```python
from build123d import *

# Parameters (mm, degrees)
SKETCH1_W          = 114.3
SKETCH1_H          = 120.65
EXTRUDE1_DEPTH     = 1.5
SKETCH2_R          = 1.55
SKETCH2_R_2        = 1.5875
CUT_EXTRUDE1_DEPTH = 84.111239463


with BuildPart() as part:
    # Sketch1 → Extrude1 (new body)
    with BuildSketch(Plane.XY):
        Rectangle(SKETCH1_W, SKETCH1_H)
    extrude(amount=EXTRUDE1_DEPTH)

    # Sketch2 → Cut-Extrude1 (cut, through all)
    with BuildSketch(Plane.XY.offset(1.5)):
        with Locations((-53.975, 3.175)):
            Circle(SKETCH2_R)
        with Locations((-47.625, -3.175)):
            Circle(SKETCH2_R)
        with Locations((53.975, 3.175)):
            Circle(SKETCH2_R)
        with Locations((47.625, -3.175)):
            Circle(SKETCH2_R)
        Circle(SKETCH2_R)
        with Locations((-53.18125, 57.15)):
            Circle(SKETCH2_R)
        with Locations((-53.18125, -19.05)):
            Circle(SKETCH2_R)
        with Locations((-53.18125, 38.1)):
            Circle(SKETCH2_R)
        with Locations((-53.18125, 19.05)):
            Circle(SKETCH2_R)
        with Locations((-53.18125, -38.1)):
            Circle(SKETCH2_R)
        with Locations((-53.18125, -57.15)):
            Circle(SKETCH2_R)
        with Locations((53.975, 57.15)):
            Circle(SKETCH2_R_2)
        with Locations((53.975, 38.1)):
            Circle(SKETCH2_R)
        with Locations((53.975, 19.05)):
            Circle(SKETCH2_R)
        with Locations((53.975, -19.05)):
            Circle(SKETCH2_R)
        with Locations((53.975, -38.1)):
            Circle(SKETCH2_R)
        with Locations((53.975, -57.15)):
            Circle(SKETCH2_R)
    extrude(amount=-CUT_EXTRUDE1_DEPTH, mode=Mode.SUBTRACT)


solid = part.part
```
The listing builds one solid part. Answer for the finished solid, in the listing's coordinates (mm). Give positions to 0.01 mm unless a question says otherwise; leave off trailing zeros. Loops run counter-clockwise (first coordinate to the right, second up) from the corner with the lowest first, then second, coordinate; pieces in that order, holes last. Notation, with made-up numbers: M -39.75,6.5 L -6.75,6.5 A23 cw -6.75,27.5 Z; hole C -35,-25 d8. An arc over 180 degrees is marked long. One line per item, written item: value.
1. Section C-C on y = -19.05 is taken. Determine the outline of the cut face in (x, z) (3 decimals).
Found:
outline: M -57.15,0 L -54.731,0 L -54.731,1.5 L -57.15,1.5 Z; M -51.631,0 L 52.425,0 L 52.425,1.5 L -51.631,1.5 Z; M 55.525,0 L 57.15,0 L 57.15,1.5 L 55.525,1.5 Z
2. Section B-B on x = 0 is taken. Determine the outline of the cut face in (y, z) (3 decimals).
Found:
outline: M -60.325,0 L -1.55,0 L -1.55,1.5 L -60.325,1.5 Z; M 1.55,0 L 60.325,0 L 60.325,1.5 L 1.55,1.5 Z
3. Section A-A on y = 57.15 is taken. Determine the outline of the cut face in (x, z).
Found:
outline: M -57.15,0 L -54.73,0 L -54.73,1.5 L -57.15,1.5 Z; M -51.63,0 L 52.39,0 L 52.39,1.5 L -51.63,1.5 Z; M 55.56,0 L 57.15,0 L 57.15,1.5 L 55.56,1.5 Z
4. Find the intervals of material crossed by probe 1 along X at (y, z) = (19, 0.85); probe 2 along X at (y, z) = (2.5, 0.2); probe 3 along Y at (x, z) = (0, 0.8) (3 decimals), in increasing order.
Found:
probe 1: -57.15 to -54.73, -51.63 to 52.43, 55.52 to 57.15
probe 2: -57.15 to -55.37, -52.58 to 52.58, 55.37 to 57.15
probe 3: -60.325 to -1.55, 1.55 to 60.325
5. For a pull along Y with two mould halves and no side action, classify faces 1 (the face through (53.639, -20.563, 0.76)), 2 (the face through (12, 1, 0)) as pulls with the +Y half, pulls with the -Y half, needs draft (parallel to the pull), parting line crosses it, or undercut.
Found:
face 1: undercut
face 2: needs draft
